Study the drawing (mm; zero at the part's minimum x, y, z) and answer. Give positions to 0.01 mm unless a question says otherwise; leave off trailing zeros. Order: outer loops, then holes, each group sorted by start corner. A loop starts at its lowest first (then second) coordinate and runs counter-clockwise, first axis right, second up. Notation, with made-up numbers: (-32.75, 22) - (23.25, 22) arc R26 ccw to (23.25, 54) - close; hole circle Ø10 at (15, 50.5). An arc over 180 degrees is marked (long way). Use CSV: the item, a comma, the result in double quotes.
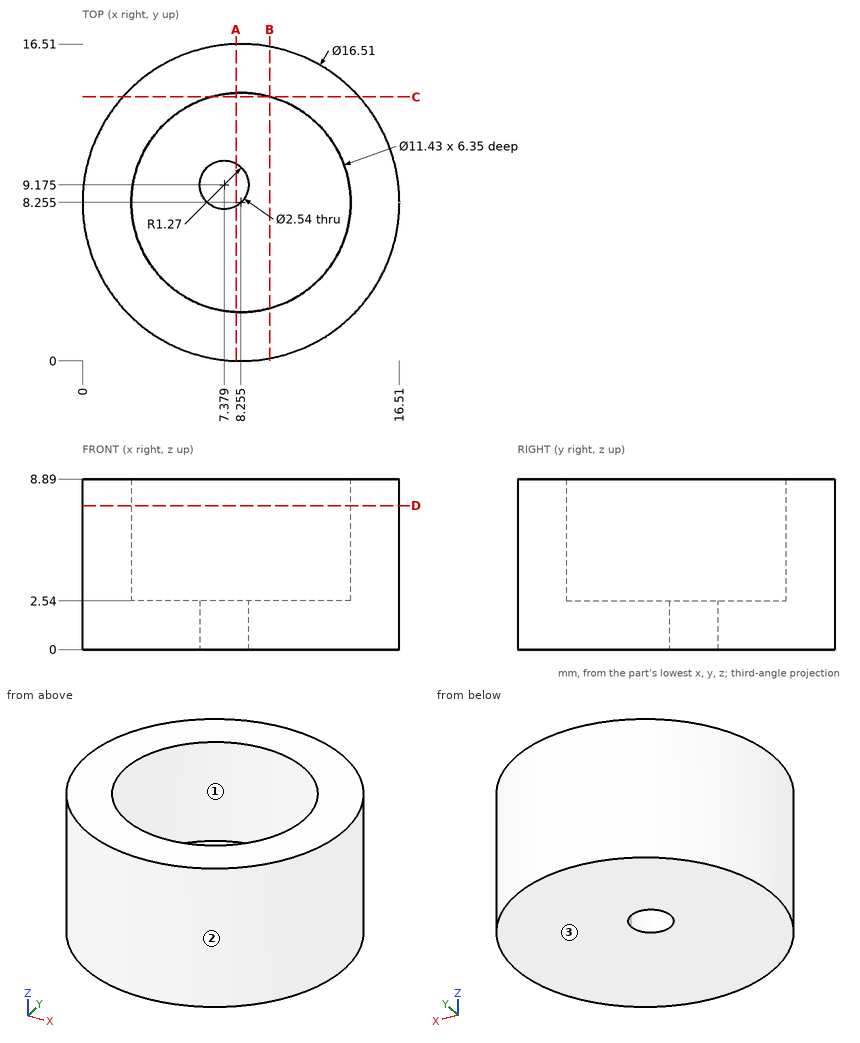
Item 1: The part is cut by section D-D (z = 7.5). Give the vertices of the cut face in (x, y) (1 decimal).
Taken from the geometry:
outline,"circle Ø16.5 at (8.3, 8.3); hole circle Ø11.4 at (8.3, 8.3)"
Item 2: Each of these flat-tipped pins is pushed along its axis until it touches: pin 1 (1.5 mm diameter, centred on y = 14, z = 3.5, fed in from +X); pin 2 (1.5 mm diameter, centred on x = 13.5, z = 3.5, fed in from -Y); pin 3 (1 mm diameter, centred on x = 11, y = 4, fed in from +Z). Where does it stop, or does it pass through?
Taken from the geometry:
pin 1,"x = 14.83"
pin 2,"y = 1.33"
pin 3,"z = 2.54"
Item 3: The part is cut by section C-C (y = 13.75). Give the vertices of the cut face in (x, z) (1 decimal).
Taken from the geometry:
outline,"(2.1, 0) - (14.4, 0) - (14.4, 8.9) - (9.8, 8.9) - (9.8, 2.5) - (6.7, 2.5) - (6.7, 8.9) - (2.1, 8.9) - close"
Item 4: The mould has two halves that part along X. Classify the marked faces 1, 2 and 3: +X half, -X half, draft (parallel to the pull), parting line (faces both ways), or undercut.
Taken from the geometry:
face 1,"undercut"
face 2,"parting line"
face 3,"draft"
Item 5: The part is cut by section B-B (x = 9.75). Give the vertices of the cut face in (y, z), and give its area (3 significant figures).
Taken from the geometry:
outline,"(0.14, 0) - (16.37, 0) - (16.37, 8.89) - (13.77, 8.89) - (13.77, 2.54) - (2.74, 2.54) - (2.74, 8.89) - (0.14, 8.89) - close"
area,"74.3 mm^2"
Item 6: The part is cut by section A-A (x = 8). Give the vertices of the cut face in (y, z) (1 decimal).
Taken from the geometry:
outline,"(0, 0) - (8.1, 0) - (8.1, 2.5) - (2.5, 2.5) - (2.5, 8.9) - (0, 8.9) - close; (10.3, 0) - (16.5, 0) - (16.5, 8.9) - (14, 8.9) - (14, 2.5) - (10.3, 2.5) - close"
Item 7: Find the intervals of material crossed by line 1 along Y through (x, z) = (7, 6) (1 decimal); line 2 along X through (y, z) = (8.5, 4.75) (1 decimal); line 3 along X through (y, z) = (9.25, 8), in increasing order.
Taken from the geometry:
line 1,"0.1 to 2.7, 13.8 to 16.4"
line 2,"0 to 2.5, 14 to 16.5"
line 3,"0.06 to 2.63, 13.88 to 16.45"
